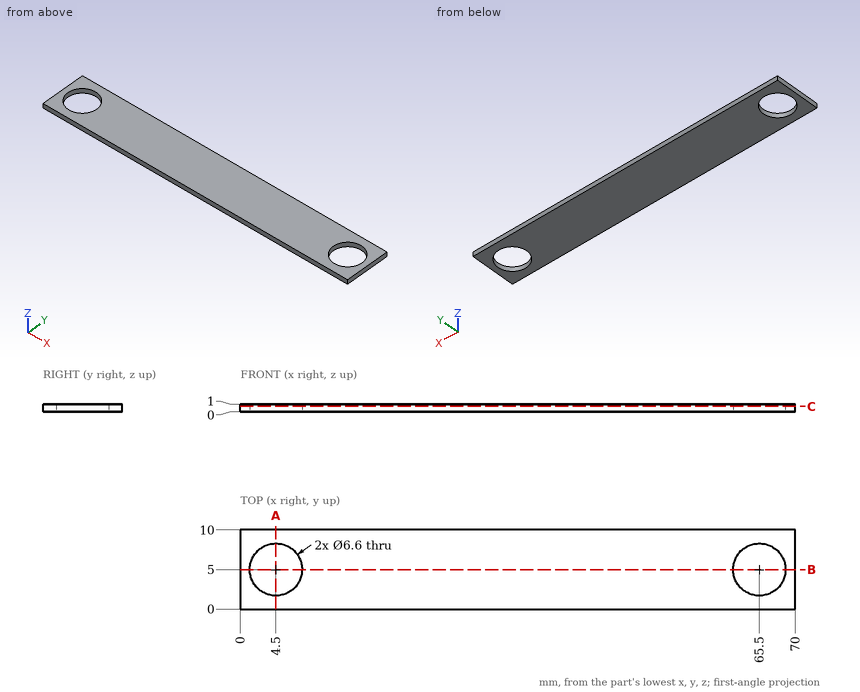
Design review of the part shown in the three views and the two pictorial views. Dimensions are in mm from the part's minimum x, y and z. Round coordinates to 2 decimals unless told otherwise and drop trailing zeros. Loops run counter-clockwise (first coordinate to the right, second up) from the corner with the lowest first, then second, coordinate; pieces in that order, holes last. Notation, with made-up numbers: (88.5, -25) - (133.5, -25) arc R20 cw to (133.5, -13) - close; hole circle Ø9 at (2.5, -29.75). An arc over 180 degrees is marked (long way). Use one line per item in the form item = value.
1) We need section A-A on x = 4.5. Write out the cut boundary in (y, z), then the cut area to 3 significant figures.
Solutions:
outline = (0, 0) - (1.7, 0) - (1.7, 1) - (0, 1) - close; (8.3, 0) - (10, 0) - (10, 1) - (8.3, 1) - close
area = 3.40 mm2
2) Clearance check with a flat-ended pin moving along its axis: P1, Ø6, axis at x = 4.5, y = 5, coming from the +Z side. State where the tip first meets the part, or that it passes through.
Solutions:
P1 = through
3) Wall thickness on probe 1 along X at (y, z) = (5, 0.7); probe 2 along Y at (x, z) = (65.5, 0.7); probe 3 along X at (y, z) = (2.5, 0.65): over which ranges is each line inside the solid? List them lowest first.
Solutions:
probe_1 = 0 to 1.2, 7.8 to 62.2, 68.8 to 70
probe_2 = 0 to 1.7, 8.3 to 10
probe_3 = 0 to 2.35, 6.65 to 63.35, 67.65 to 70
4) We need section B-B on y = 5. Write out the cut boundary in (x, z), then the cut area to 3 significant figures.
Solutions:
outline = (0, 0) - (1.2, 0) - (1.2, 1) - (0, 1) - close; (7.8, 0) - (62.2, 0) - (62.2, 1) - (7.8, 1) - close; (68.8, 0) - (70, 0) - (70, 1) - (68.8, 1) - close
area = 56.8 mm2
5) We need section C-C on z = 0.7. Write out the cut boundary in (x, y), then the cut area to 3 significant figures.
Solutions:
outline = (0, 0) - (70, 0) - (70, 10) - (0, 10) - close; hole circle Ø6.6 at (4.5, 5); hole circle Ø6.6 at (65.5, 5)
area = 632 mm2
